For this review, take the finished solid that the model builds, in its own axes (mm). A direction names the side the tool comes from. Give positions to 0.01 mm unless a question says otherwise; leave off trailing zeros. Write each loop counter-clockwise with the first axis right and the second up, starting at its lowest first coordinate (ties: lowest second). Pieces come first, ordered by that corner, then holes.
Q1. We need section B-B (z = -16.5). Write out the cut boundary in (x, y), then the cut area to 3 significant figures.
Q2. We need section C-C (y = -7.5). Write out the cut boundary in (x, z).
Q3. Mouldability with a two-part tool opening along X and no side actions: class faces 1 (the cylindrical face through (-4.88, -4.93, 37.18)), 2 (the cylindrical face through (14.246, 0.14, 22.345)), 3 (the flat face through (28, 0, -30)), 4 (the flat face through (37.5, 5, 1)) as released by +X, released by -X, zero draft, split by the parting line, or undercut.
Q4. We need section A-A (x = 15.5). Write out the cut boundary in (y, z).
Q5. Machinability: for faces 5 (the flat face through (-30, 0, -29)), 6 (the flat face through (-30, 0, 28)), 7 (the flat face through (30, 0, 30)), which of the approach directions +Z, -Z, +X, -X, +Y, -Y give a long, thin tool a straight path to every point of the face, cutting with its end or side? Answer none if there is none.
Q6. For line 1 (Z direction, x = 1, y = 6.5); line 2 (X direction, y = 4.75, z = 0); line 3 (Y direction, x = 29, z = -29.5), list the stretches that pass through material, from the lowest coordinate up.
Q7. Insertion check: P1, Ø4, axis at x = 9.5, y = -6.5, coming from the -Z side; P2, Ø1, axis at y = -7, z = 3.5, coming from the +X side; P3, Ø1.5, axis at y = -3, z = -22, coming from the -X side. Each pin has a flat end and moves straight along its axis. Give the tip position at first contact, or say it passes through.
Q8. We need section D-D (y = 3.5). Write out the cut boundary in (x, z), then the cut area to 3 significant figures.
```python
from build123d import *

# Parameters (mm, degrees)
SKETCH1_W           = 75
SKETCH1_H           = 75
SKETCH1_R           = 26.5
BOSS_EXTRUDE1_DEPTH = 10
SKETCH2_R           = 37.5
SKETCH2_R_2         = 26.5
BOSS_EXTRUDE2_DEPTH = 10


with BuildPart() as part:
    # Sketch1 → Boss-Extrude1 (new body)
    with BuildSketch(Plane(origin=(0, 0, 0), x_dir=(1, 0, 0), z_dir=(0, 1, 0))):
        Rectangle(SKETCH1_W, SKETCH1_H)
        Circle(SKETCH1_R, mode=Mode.SUBTRACT)
    extrude(amount=BOSS_EXTRUDE1_DEPTH)

    # Sketch2 → Boss-Extrude2 (add)
    with BuildSketch(Plane.XZ):
        Circle(SKETCH2_R)
        Circle(SKETCH2_R_2, mode=Mode.SUBTRACT)
    extrude(amount=BOSS_EXTRUDE2_DEPTH)


solid = part.part
```
Computed:
1. outline: (-37.5, 0) - (-33.67, 0) - (-33.67, -10) - (-20.74, -10) - (-20.74, 10) - (-37.5, 10) - close; (20.74, -10) - (33.67, -10) - (33.67, 0) - (37.5, 0) - (37.5, 10) - (20.74, 10) - close
1. area: 594 mm2
2. outline: circle Ø75 at (0, 0); hole circle Ø53 at (0, 0)
3. face 1: split by the parting line
3. face 2: undercut
3. face 3: zero draft
3. face 4: released by +X
4. outline: (-10, -34.15) - (0, -34.15) - (0, -37.5) - (10, -37.5) - (10, -21.49) - (-10, -21.49) - close; (-10, 21.49) - (10, 21.49) - (10, 37.5) - (0, 37.5) - (0, 34.15) - (-10, 34.15) - close
5. face 5: -Z, -X, -Y
5. face 6: +Z, -X, -Y
5. face 7: +Z, +X, -Y
6. line 1: z = -37.5 to -26.48, 26.48 to 37.5
6. line 2: x = -37.5 to -26.5, 26.5 to 37.5
6. line 3: y = 0 to 10
7. P1: stops at z = -36.74
7. P2: stops at x = 37.38
7. P3: stops at x = -30.9
8. outline: (-37.5, -37.5) - (37.5, -37.5) - (37.5, 37.5) - (-37.5, 37.5) - close; hole circle Ø53 at (0, 0)
8. area: 3,420 mm2
